The listing builds one solid part. Answer for the finished solid, in the listing's coordinates (mm). Round coordinates to 2 decimals unless told otherwise and drop trailing zeros. Write each loop counter-clockwise with the first axis right and the second up, starting at its lowest first coordinate (ties: lowest second). Pieces come first, ordered by that corner, then holes. Notation, with made-up numbers: (89.5, -20.75) - (124.5, -20.75) arc R19 ccw to (124.5, -13.75) - close; hole circle Ø7 at (-21.5, 54.25). An arc over 180 degrees is marked (long way). Answer in a Markdown table with one row per item.
from build123d import *

# Parameters (mm, degrees)
F2_DEPTH = 1910
F7_DEPTH = 700
F9_DEPTH = 2000


with BuildPart() as f2:
    # F1 (on Front) → F2 (new body)
    with BuildSketch(Plane.XZ):
        with BuildLine():
            Line((7.5, 37.974085065), (7.5, 40))
            Line((7.5, 40), (-15, 40))
            Line((-15, 40), (-15, 37))
            Line((-15, 37), (-15, 31))
            Line((-15, 31), (-15, 29))
            Line((-15, 29), (-15, 26))
            Line((-15, 26), (-15, 24))
            Line((-15, 24), (-13, 24))
            Line((-13, 24), (-11, 24))
            Line((-11, 24), (-11, 26))
            Line((-11, 26), (-9, 26))
            Line((-9, 26), (-9, 20))
            Line((-9, 20), (-11, 20))
            Line((-11, 20), (-11, 22))
            Line((-11, 22), (-15, 22))
            Line((-15, 22), (-15, 18))
            Line((-15, 18), (-15, 7.7))
            Line((-15, 7.7), (-13, 7.7))
            Line((-13, 7.7), (-13, 11.4920835048))
            Line((-13, 11.4920835048), (-7, 11.4920835048))
            Line((-7, 11.4920835048), (-7, 3.7))
            Line((-7, 3.7), (-11, 3.7))
            Line((-11, 3.7), (-11, 5.7))
            Line((-11, 5.7), (-15, 5.7))
            Line((-15, 5.7), (-15, 3))
            Line((-15, 3), (-15, 0))
            Line((-15, 0), (-13, 0))
            Line((-13, 0), (-12, 0))
            Line((-12, 0), (-5, 0))
            Line((-5, 0), (-5, 13.4920835048))
            Line((-5, 13.4920835048), (-7, 13.4920835048))
            Line((-7, 13.4920835048), (-9.1588944197, 13.4920835048))
            Line((-9.1588944197, 13.4920835048), (-9.1588944197, 15.4920835048))
            Line((-9.1588944197, 15.4920835048), (1.5, 20))
            Line((1.5, 20), (10.8411055803, 15.4920835048))
            Line((10.8411055803, 15.4920835048), (10.8411055803, 13.4920835048))
            Line((10.8411055803, 13.4920835048), (8, 13.4920835048))
            Line((8, 13.4920835048), (8, 0))
            Line((8, 0), (17, 0))
            Line((17, 0), (17, 40))
            Line((17, 40), (8.5, 40))
            Line((8.5, 40), (8.5, 37.974085065))
            ThreePointArc((8.5, 37.974085065), (11.5604089792, 36.6859489396), (13.3185590744, 33.8691589154))
            Line((13.3185590744, 33.8691589154), (13.4318527537, 31.7073867348))
            ThreePointArc((13.4318527537, 31.7073867348), (4.0126863822, 28.7323088758), (7.5, 37.974085065))
        make_face()
        Polygon((-8.3634709733, 18), (-11.1588944197, 16.817744602), (-11.1588944197, 15.4920835048), (-11.1588944197, 13.4920835048), (-13, 13.4920835048), (-13, 18), align=None, mode=Mode.SUBTRACT)
        with BuildLine():
            Line((-13, 34), (-13, 37.9999987781))
            Line((-13, 37.9999987781), (2.9081163149, 37.9999987781))
            ThreePointArc((2.9081163149, 37.9999987781), (3.810445381, 26.2974906682), (15, 29.8410427327))
            Line((15, 29.8410427327), (15, 2))
            Line((15, 2), (10, 2))
            Line((10, 2), (10, 12))
            Line((10, 12), (12.8411055803, 12))
            Line((12.8411055803, 12), (12.8411055803, 16.7476188273))
            Line((12.8411055803, 16.7476188273), (1.5543358685, 22.194491783))
            Line((1.5543358685, 22.194491783), (-7, 18.5766464184))
            Line((-7, 18.5766464184), (-7, 28))
            Line((-7, 28), (-13, 28))
            Line((-13, 28), (-13, 34))
        make_face(mode=Mode.SUBTRACT)
        with BuildLine():
            Line((13.0918836851, 37.9999987781), (13.1020709306, 37.9999987781))
            Line((13.1020709306, 37.9999987781), (13.1025921338, 37.9900536295))
            ThreePointArc((13.1025921338, 37.9900536295), (13.0972403349, 37.9950288154), (13.0918836851, 37.9999987781))
        make_face(mode=Mode.SUBTRACT)
    extrude(amount=-F2_DEPTH)

    # F8 (on face) → F9 (cut)
    with BuildSketch(Plane.XZ):
        Polygon((17, 0), (17, 40), (-15, 40), (-15, 3), (-15, 0), align=None)
    extrude(amount=-F9_DEPTH, mode=Mode.SUBTRACT)


with BuildPart() as f7:
    # F6 (on face) → F7 (new body)
    with BuildSketch(Plane.XZ):
        with BuildLine():
            ThreePointArc((-25.5, 37.9771982231), (-25.951759356, 27.0133522571), (-26.596, 37.9675733099))
            Line((-26.596, 37.9675733099), (-26.596, 40))
            Line((-26.596, 40), (-49.096, 40))
            Line((-49.096, 40), (-49.096, 18))
            Line((-49.096, 18), (-17, 18))
            Line((-17, 18), (-17, 22))
            Line((-17, 22), (-19, 22))
            Line((-19, 22), (-19, 20))
            Line((-19, 20), (-47.096, 20))
            Line((-47.096, 20), (-47.096, 38))
            Line((-47.096, 38), (-31.0964418097, 38))
            ThreePointArc((-31.0964418097, 38), (-30.1932729017, 26.2962600635), (-19, 29.8323432536))
            Line((-19, 29.8323432536), (-19, 24))
            Line((-19, 24), (-17, 24))
            Line((-17, 24), (-17, 40))
            Line((-17, 40), (-25.5, 40))
            Line((-25.5, 40), (-25.5, 37.9771982231))
        make_face()
    extrude(amount=-F7_DEPTH)


solid = f7.part
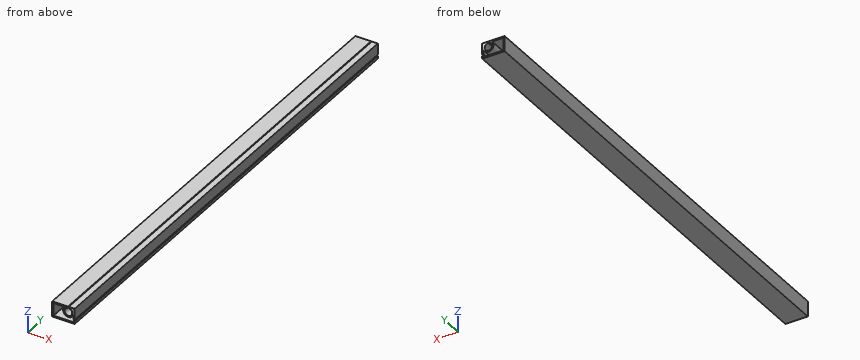
(1) Find the intervals of material crossed by line 1 (Z direction, x = -41.5, y = 565); line 2 (X direction, y = 50, z = 35.5); line 3 (Z direction, x = -23, y = 411.5), in increasing order.
Checked values:
| item | result |
|---|---|
| line 1 | z = 18 to 20, 38 to 40 |
| line 2 | x = -49.1 to -47.1, -32.87 to -30.61, -21.39 to -17 |
| line 3 | z = 18 to 20, 25.64 to 27.9, 37.11 to 40 |
(2) Section B-B (y = 478.5) is taken. Give the vertices of the cut face in (x, z), and give its area (3 significant figures).
Checked values:
| item | result |
|---|---|
| outline | (-49.1, 18) - (-17, 18) - (-17, 22) - (-19, 22) - (-19, 20) - (-47.1, 20) - (-47.1, 38) - (-31.1, 38) arc R7.49 ccw (long way) to (-19, 29.83) - (-19, 24) - (-17, 24) - (-17, 40) - (-25.5, 40) - (-25.5, 37.98) arc R5.49 cw (long way) to (-26.6, 37.97) - (-26.6, 40) - (-49.1, 40) - close |
| area | 262 mm2 |
(3) A flat-ended cylindrical pin translates along its axis: pin 1 (2 mm diameter, centred on x = -21.5, z = 24.5, fed in from -Y). Find the tip coordinate at first contact, or state that the pin passes through.
Checked values:
| item | result |
|---|---|
| pin 1 | passes through |
(4) Section A-A (x = -40.5) is taken. Give the vertices of the cut face in (y, z), and give its area (3 significant figures).
Checked values:
| item | result |
|---|---|
| outline | (0, 18) - (700, 18) - (700, 20) - (0, 20) - close; (0, 38) - (700, 38) - (700, 40) - (0, 40) - close |
| area | 2,800 mm2 |
